from build123d import *

# Parameters (mm, degrees)
F3_R      = 80
F4_DEPTH  = 35
F5_R      = 67.5
F6_DEPTH  = 33
F7_R      = 55
F8_DEPTH  = 33
F9_R      = 48
F10_DEPTH = 64
F11_R     = 22
F12_R     = 17.5
F14_R     = 74
F15_DEPTH = 27
F16_R     = 61
F17_DEPTH = 60.001
F18_R     = 22
F19_R     = 17.5
F21_R     = 11.11
F22_DEPTH = 133.0010001
F24_R     = 3


# Not quite as in the source:
# - a fillet or chamfer that OpenCascade refuses, or shapes differently, is made with other operations: its cross-section is extruded or revolved along the edge and cut away or added


with BuildPart() as f4:
    # F3 (on Front) → F4 (new body)
    with BuildSketch(Plane.XZ):
        Circle(F3_R)
    extrude(amount=F4_DEPTH)

    # F5 (on face) → F6 (join)
    with BuildSketch(Plane.XZ.offset(35)):
        with Locations((-1.0126e-06, -0.7260435959)):
            Circle(F5_R)
    extrude(amount=F6_DEPTH)

    # F7 (on face) → F8 (join)
    with BuildSketch(Plane.XZ.offset(68)):
        Circle(F7_R)
    extrude(amount=F8_DEPTH)

    # F9 (on offset) → F10 (cut)
    with BuildSketch(Plane.XZ.offset(133)):
        Circle(F9_R)
    extrude(amount=-F10_DEPTH, mode=Mode.SUBTRACT)

    # F11 (on face) → F13 section 0
    with BuildSketch(Plane.XZ.offset(69)):
        Circle(F11_R)
    # F12 (on offset) → F13 section 1
    with BuildSketch(Plane.XZ.offset(133)):
        Circle(F12_R)
    loft()

    # F14 (on Front) → F15 (cut)
    with BuildSketch(Plane.XZ):
        Circle(F14_R)
    extrude(amount=F15_DEPTH, mode=Mode.SUBTRACT)

    # F16 (on offset) → F17 (cut, through all)
    with BuildSketch(Plane.XZ.offset(60)):
        with Locations((0, -3.5063521937)):
            Circle(F16_R)
    extrude(amount=-F17_DEPTH, mode=Mode.SUBTRACT)

    # F18 (on face) → F20 section 0
    with BuildSketch(Plane(origin=(0, -60, 0), x_dir=(-1, 0, 0), z_dir=(0, 1, 0))):
        Circle(F18_R)
    # F19 (on offset) → F20 section 1
    with BuildSketch(Plane.XZ.offset(28)):
        Circle(F19_R)
    loft()

    # F21 (on Front) → F22 (cut, through all)
    with BuildSketch(Plane.XZ):
        Circle(F21_R)
    extrude(amount=F22_DEPTH, mode=Mode.SUBTRACT)

    # F23: chamfer of 2 on 2 edges, made by hand

    # F23_s1 → F23_t2 (revolve, cut)
    with BuildSketch(Plane.XY):
        Polygon((50, -101), (48, -99), (48, -101), align=None)
    revolve(axis=Axis((0, -101, 0), (0, -1, 0)), mode=Mode.SUBTRACT)

    # F23_s3 → F23_t4 (revolve, cut)
    with BuildSketch(Plane.XY):
        Polygon((17.6307616561, -131.1402786693), (15.6356872477, -133), (17.5, -133), align=None)
    revolve(axis=Axis((0, -133, 0), (0, -1, 0)), mode=Mode.SUBTRACT)

    # F24
    f24_edges = [f4.edges().sort_by_distance(p)[0] for p in [
        (-22, -69, 0),
        (-48, -69, 0),
        (-61, -60, -3.506352),
        (22, -60, 0),
    ]]
    fillet(f24_edges, radius=F24_R)


solid = f4.part
The model under review builds one solid part; all positions refer to its coordinate system, in mm. A direction names the side the tool comes from. Round coordinates to 2 decimals unless told otherwise and drop trailing zeros. Loops run counter-clockwise (first coordinate to the right, second up) from the corner with the lowest first, then second, coordinate; pieces in that order, holes last. Notation, with made-up numbers: (-26.5, -22.75) -> (-8.5, -22.75) arc R25 cw to (-8.5, -7.75) -> close; hole circle Ø1 at (2, -15.5). An arc over 180 degrees is marked (long way). One line per question, with ' | ' between items. Start each with the question number.
Item 1: Add section C-C, the plane y = -17. Write out the cut boundary in (x, z).
Item 2: Add section D-D, the plane y = -116.5. Write out the cut boundary in (x, z), then the cut area to 3 significant figures.
Item 3: Wall thickness on line 1 along Z through (x, y) = (0, -80.5); line 2 along Z through (x, y) = (0.5, -22.5); line 3 along Z through (x, y) = (0, -43): over which ranges is each line inside the solid? List them lowest first. Write a range as [from, to].
Item 4: For pin 1 (1 mm diameter, centred on y = -92.5, z = -22, fed in from +X); pin 2 (10 mm diameter, centred on x = -22.5, y = -45, fed in from +Z); pin 3 (8 mm diameter, centred on x = -19, z = 28, fed in from +Y), all flat-tipped, find the tip position at first contact; note any pin that passes through.
Item 5: Add section B-B, the plane z = 64. Write out the cut boundary in (x, y), then the cut area to 3 significant figures.
Item 6: Machinability: for faces 4 (the face through (22, -27, 55)), 5 (the face through (-11.923, -84.269, -53.692)), 6 (the face through (23, 0, -71)), which of the approach directions +Z, -Z, +X, -X, +Y, -Y give a long, thin tool a straight path to every point of the face, cutting with its end or side? Answer none if there is none.
Item 7: Draft analysis for pull direction Z (two halves, no side actions). For faces 1 (the face through (12, -101, -49)), 2 (the face through (-47.954, -85.689, 2.11)), 3 (the face through (-17.34, -17.26, -78.1)), state which applies: +Z half, -Z half, draft (parallel to the pull), parting line (faces both ways), or undercut.
Item 8: Add section A-A, the plane y = -85. Write out the cut boundary in (x, z) (3 decimals), then the cut area to 3 significant figures.
Return value:
1) outline: circle Ø160 at (0, 0); hole circle Ø148 at (0, 0)
2) outline: circle Ø37.32 at (0, 0); hole circle Ø22.22 at (0, 0) | area: 706 mm2
3) line 1: z = [-55, -48], [-21.19, -11.11], [11.11, 21.19], [48, 55] | line 2: z = [-80, -74], [74, 80] | line 3: z = [-68.23, -64.51], [-19.61, -11.11], [11.11, 19.61], [57.49, 66.77]
4) pin 1: stops at x = 50.62 | pin 2: stops at z = 64.47 | pin 3: stops at y = -60
5) outline: (-48, -35) -> (-19.15, -35) -> (-19.15, -68) -> (19.15, -68) -> (19.15, -35) -> (48, -35) -> (48, 0) -> (37.15, 0) -> (37.15, -27) -> (-37.15, -27) -> (-37.15, 0) -> (-48, 0) -> close | area: 2,620 mm2
6) face 4: +Y | face 5: -Y | face 6: +Z, -Z, +X, -X, +Y
7) face 1: draft | face 2: undercut | face 3: parting line
8) outline: circle Ø110 at (0, 0); circle Ø41.75 at (0, 0); hole circle Ø96 at (0, 0); hole circle Ø22.22 at (0, 0) | area: 3,250 mm2
